CAD build for the part. Positions are in the model's coordinates, mm. Give positions to 0.01 mm unless a question says otherwise; leave off trailing zeros. Write each loop counter-clockwise with the first axis right and the second up, starting at its lowest first coordinate (ties: lowest second). Pieces come first, ordered by that corner, then holes. Notation, with made-up numbers: (64.25, 48) -> (88.25, 48) arc R23 cw to (88.25, 83) -> close; hole circle Ø8 at (39, -7). An arc over 180 degrees is marked (long way). Answer in a Markdown table with one row per item. Add a question column.
```python
from build123d import *

# Parameters (mm, degrees)
EXTRUDE_1_DEPTH     = 2
SKETCH_3_W          = 180
SKETCH_3_H          = 35
EXTRUDE_2_DEPTH     = 2
SKETCH_4_W          = 180
SKETCH_4_H          = 20
EXTRUDE_3_DEPTH     = 2
SKETCH_5_W          = 140
SKETCH_5_H          = 87
CUT_EXTRUDE_1_DEPTH = 194.062166154
FILLET_1_R          = 10
FILLET_2_R          = 10
FILLET_3_R          = 10
FILLET_4_R          = 10
CUT_EXTRUDE_2_DEPTH = 10
FILLET_5_R          = 10
FILLET_6_R          = 10
CUT_EXTRUDE_5_DEPTH = 10
CUT_EXTRUDE_6_DEPTH = 194.062166154
CUT_EXTRUDE_7_DEPTH = 194.062166154
SKETCH_13_R         = 1.6
CUT_EXTRUDE_8_DEPTH = 10


with BuildPart() as part:
    # 草图2 → 凸台-拉伸1 (new body)
    with BuildSketch(Plane.XY):
        Polygon((90, 100), (90, 39), (138, 39), (138, -35), (90, -35), (90, -100), (-90, -100), (-90, -35), (-138, -35), (-138, 39), (-90, 39), (-90, 100), align=None)
    extrude(amount=EXTRUDE_1_DEPTH)

    # 草图3 → 凸台-拉伸2 (add)
    with BuildSketch(Plane.XY.offset(2)):
        with Locations((0, -117.5)):
            Rectangle(SKETCH_3_W, SKETCH_3_H)
    extrude(amount=-EXTRUDE_2_DEPTH)

    # 草图4 → 凸台-拉伸3 (add)
    with BuildSketch(Plane.XY.offset(2)):
        with Locations((0, 110)):
            Rectangle(SKETCH_4_W, SKETCH_4_H)
    extrude(amount=-EXTRUDE_3_DEPTH)

    # 草图5 → 切除-拉伸1 (cut, through all)
    with BuildSketch(Plane(origin=(0, 0, 0), x_dir=(-1, 0, 0), z_dir=(0, 0, -1))):
        with Locations((0, -11.5)):
            Rectangle(SKETCH_5_W, SKETCH_5_H)
    extrude(amount=-CUT_EXTRUDE_1_DEPTH, mode=Mode.SUBTRACT)

    # 圆角1
    fillet_1_edges = [part.edges().sort_by_distance(p)[0] for p in [
        (138, -35, 1),
    ]]
    fillet(fillet_1_edges, radius=FILLET_1_R)

    # 圆角2
    fillet_2_edges = [part.edges().sort_by_distance(p)[0] for p in [
        (138, 39, 1),
    ]]
    fillet(fillet_2_edges, radius=FILLET_2_R)

    # 圆角3
    fillet_3_edges = [part.edges().sort_by_distance(p)[0] for p in [
        (-138, 39, 1),
    ]]
    fillet(fillet_3_edges, radius=FILLET_3_R)

    # 圆角4
    fillet_4_edges = [part.edges().sort_by_distance(p)[0] for p in [
        (-138, -35, 1),
    ]]
    fillet(fillet_4_edges, radius=FILLET_4_R)

    # 草图7 → 切除-拉伸2 (cut)
    with BuildSketch(Plane(origin=(0, 0, 0), x_dir=(-1, 0, 0), z_dir=(0, 0, -1))):
        with BuildLine():
            Line((-70, 115.6), (70, 115.6))
            ThreePointArc((70, 115.6), (71.6, 114), (70, 112.4))
            Line((70, 112.4), (-70, 112.4))
            ThreePointArc((-70, 112.4), (-71.6, 114), (-70, 115.6))
        make_face()
        with BuildLine():
            Line((-70, 102.6), (70, 102.6))
            ThreePointArc((70, 102.6), (71.6, 101), (70, 99.4))
            Line((70, 99.4), (-70, 99.4))
            ThreePointArc((-70, 99.4), (-71.6, 101), (-70, 102.6))
        make_face()
        with BuildLine():
            Line((-70, 39.6), (70, 39.6))
            ThreePointArc((70, 39.6), (71.6, 38), (70, 36.4))
            Line((70, 36.4), (-70, 36.4))
            ThreePointArc((-70, 36.4), (-71.6, 38), (-70, 39.6))
        make_face()
    extrude(amount=-CUT_EXTRUDE_2_DEPTH, mode=Mode.SUBTRACT)

    # 圆角5
    fillet_5_edges = [part.edges().sort_by_distance(p)[0] for p in [
        (-90, 120, 1),
    ]]
    fillet(fillet_5_edges, radius=FILLET_5_R)

    # 圆角6
    fillet_6_edges = [part.edges().sort_by_distance(p)[0] for p in [
        (90, 120, 1),
    ]]
    fillet(fillet_6_edges, radius=FILLET_6_R)

    # 草图10 → 切除-拉伸5 (cut)
    with BuildSketch(Plane(origin=(0, 0, 0), x_dir=(-1, 0, 0), z_dir=(0, 0, -1))):
        with BuildLine():
            Line((-70, -61.3), (70, -61.3))
            ThreePointArc((70, -61.3), (71.6, -62.9), (70, -64.5))
            Line((70, -64.5), (-70, -64.5))
            ThreePointArc((-70, -64.5), (-71.6, -62.9), (-70, -61.3))
        make_face()
        with BuildLine():
            Line((-70, -119.4), (70, -119.4))
            ThreePointArc((70, -119.4), (71.6, -121), (70, -122.6))
            Line((70, -122.6), (-70, -122.6))
            ThreePointArc((-70, -122.6), (-71.6, -121), (-70, -119.4))
        make_face()
    extrude(amount=-CUT_EXTRUDE_5_DEPTH, mode=Mode.SUBTRACT)

    # 草图11 → 切除-拉伸6 (cut, through all)
    with BuildSketch(Plane.XY.offset(2)):
        with BuildLine():
            Line((-65, 88.7), (65, 88.7))
            ThreePointArc((65, 88.7), (66.6, 87.1), (65, 85.5))
            Line((65, 85.5), (-65, 85.5))
            ThreePointArc((-65, 85.5), (-66.6, 87.1), (-65, 88.7))
        make_face()
    extrude(amount=-CUT_EXTRUDE_6_DEPTH, mode=Mode.SUBTRACT)

    # 草图12 → 切除-拉伸7 (cut, through all)
    with BuildSketch(Plane.XY.offset(2)):
        with BuildLine():
            Line((81.6, 12), (81.6, -33))
            ThreePointArc((81.6, -33), (80, -34.6), (78.4, -33))
            Line((78.4, -33), (78.4, 12))
            ThreePointArc((78.4, 12), (80, 13.6), (81.6, 12))
        make_face()
        with BuildLine():
            Line((-81.6, 12), (-81.6, -33))
            ThreePointArc((-81.6, -33), (-80, -34.6), (-78.4, -33))
            Line((-78.4, -33), (-78.4, 12))
            ThreePointArc((-78.4, 12), (-80, 13.6), (-81.6, 12))
        make_face()
    extrude(amount=-CUT_EXTRUDE_7_DEPTH, mode=Mode.SUBTRACT)

    # 草图13 → 切除-拉伸8 (cut)
    with BuildSketch(Plane.XY.offset(2)):
        with Locations((-72.5, 82.5)):
            Circle(SKETCH_13_R)
        with Locations((-72.5, 42.5)):
            Circle(SKETCH_13_R)
        with Locations((72.5, 82.5)):
            Circle(SKETCH_13_R)
        with Locations((72.5, 42.5)):
            Circle(SKETCH_13_R)
    extrude(amount=-CUT_EXTRUDE_8_DEPTH, mode=Mode.SUBTRACT)


solid = part.part
```
Item 1: Drop flat-ended pins along their axis: pin 1 Ø2.5 at (x, y) = (72.5, 82.5) entering from -Z; pin 2 Ø1 at (y, z) = (70.5, 0.5) entering from +X; pin 3 Ø1 at (y, z) = (81.5, 1.5) entering from -X. Give the stop position or say it passes through.
Item 2: Probe L1, parallel to Y at x = 72.5, z = 0.85; L2, parallel to X at y = -3.5, z = 1.9; L3, parallel to X at y = 30, z = 0.75. List the from-to ranges inside material, lowest first. Write a range as from..to.
Item 3: Slice it at A-A, the plane x = 2. State how many separate pieces and enclosed holes the cut face has, then the cut area to 3 significant figures.
Item 4: Slice it at B-B, the plane y = -16. List the corners of the cut face in (x, z), then the cut area to 3 significant figures.
Item 5: Slice it at D-D, the plane x = -111. List the corners of the cut face in (y, z).
Answer key:
| question | item | result |
|---|---|---|
| 1 | pin 1 | passes through |
| 1 | pin 2 | stops at x = 90 |
| 1 | pin 3 | stops at x = -90 |
| 2 | L1 | y = -135..40.9, 44.1..80.9, 84.1..120 |
| 2 | L2 | x = -138..-81.6, -78.4..-70, 70..78.4, 81.6..138 |
| 2 | L3 | x = -137.95..-70, 70..137.95 |
| 3 | separate pieces | 8 |
| 3 | enclosed holes | 0 |
| 3 | area | 298 mm² |
| 4 | outline | (-138, 0) -> (-81.6, 0) -> (-81.6, 2) -> (-138, 2) -> close; (-78.4, 0) -> (-70, 0) -> (-70, 2) -> (-78.4, 2) -> close; (70, 0) -> (78.4, 0) -> (78.4, 2) -> (70, 2) -> close; (81.6, 0) -> (138, 0) -> (138, 2) -> (81.6, 2) -> close |
| 4 | area | 259 mm² |
| 5 | outline | (-35, 0) -> (39, 0) -> (39, 2) -> (-35, 2) -> close |
